Here's how the part is built. I have some questions about the finished solid (model axes, mm). A direction names the side the tool comes from. Coordinates: 2 decimals unless noted, no trailing zeros. Loops run counter-clockwise (first coordinate to the right, second up) from the corner with the lowest first, then second, coordinate; pieces in that order, holes last. Notation, with made-up numbers: (5.5, 0) - (16.5, 0) arc R12 cw to (16.5, 12) - close; hole circle Ø10 at (30.5, 33.5). An arc over 180 degrees is marked (long way). Use a Markdown table: item, result.
```python
from build123d import *

# Parameters (mm, degrees)
F0_W     = 90
F0_H     = 4
F1_DEPTH = 5
F2_R     = 1.661067913
F3_DEPTH = 3.5
F6_W     = 1.3
F6_H     = 4
F7_DEPTH = 1.3
F8_W     = 3.1040143222
F8_H     = 3.8397812168
F9_DEPTH = 89


# Not quite as in the source:
# - the program builds the solid bodies; features that only make, move or delete a surface that nothing else refers to are left out


with BuildPart() as f1:
    # F0 (on Top) → F1 (new body)
    with BuildSketch(Plane.XY):
        with Locations((9.9665279686, 16.8302931339)):
            Rectangle(F0_W, F0_H)
    extrude(amount=F1_DEPTH)

    # F2 (on face) → F3 (cut)
    with BuildSketch(Plane.XY.offset(5)):
        with Locations((-33.0299064517, 16.7948473245)):
            Circle(F2_R)
    extrude(amount=-F3_DEPTH, mode=Mode.SUBTRACT)

    # F6 (on face) → F7 (cut)
    with BuildSketch(Plane(origin=(0, 0, 0), x_dir=(1, 0, 0), z_dir=(0, 0, -1))):
        with Locations((6.5131389402, -16.8302931339)):
            Rectangle(F6_W, F6_H)
    extrude(amount=-F7_DEPTH, mode=Mode.SUBTRACT)

    # F8 (on face) → F9 (cut)
    with BuildSketch(Plane.YZ.offset(54.9665279686)):
        with Locations((16.8456220999, 2.3313869315)):
            Rectangle(F8_W, F8_H)
    extrude(amount=-F9_DEPTH, mode=Mode.SUBTRACT)


solid = f1.part
```
Q1. Please list where these lines run through material, in increasing order: L1, parallel to Z at x = 4, y = 16.2; L2, parallel to X at y = 17.6, z = 0.35; L3, parallel to Y at x = -11, z = 4.05. Write a range as from..to.
Check values:
| item | result |
|---|---|
| L1 | 0..0.41, 4.25..5 |
| L2 | -35.03..5.86, 7.16..54.97 |
| L3 | 14.83..15.29, 18.4..18.83 |
Q2. I want a section at B-B, the plane z = 2.4. Write out the boundary of the cut face in (x, y).
Check values:
| item | result |
|---|---|
| outline | (-35.03, 14.83) - (54.97, 14.83) - (54.97, 15.29) - (-32.32, 15.29) arc R1.66 cw to (-33.74, 15.29) - (-34.03, 15.29) - (-34.03, 15.47) arc R1.66 cw to (-34.03, 18.12) - (-34.03, 18.4) - (-33.47, 18.4) arc R1.66 cw to (-32.59, 18.4) - (54.97, 18.4) - (54.97, 18.83) - (-35.03, 18.83) - close |
Q3. Which directions (+Z, -Z, +X, -X, +Y, -Y) give clear straight access to the entire face, cutting with the end or side of a thin tool? Please do faces 4 (the face through (-14, 17, 0.411)), 5 (the face through (-35.033, 17, 2)).
Check values:
| item | result |
|---|---|
| face 4 | +X |
| face 5 | +Z, -Z, -X, +Y, -Y |
Q4. Will this pin go through, and if not, where does the flat tip stop? P1, Ø0.5, axis at x = -34.5, y = 16.5, coming from the +Z side.
Check values:
| item | result |
|---|---|
| P1 | z = 5 |
Q5. I want a section at A-A, the plane x = -6. Write out the boundary of the cut face in (y, z).
Check values:
| item | result |
|---|---|
| outline | (14.83, 0) - (18.83, 0) - (18.83, 5) - (14.83, 5) - close; hole (15.29, 0.41) - (18.4, 0.41) - (18.4, 4.25) - (15.29, 4.25) - close |
Q6. If we mould it in two halves opening along X, with no side actions, what happens to faces 1 (the face through (-34.033, 17, 1)), 2 (the face through (12, 17, 4.251)), 3 (the face through (-34.69, 16.87, 3.66))? For each: pulls with the +X half, pulls with the -X half, needs draft (parallel to the pull), parting line crosses it, or undercut.
Check values:
| item | result |
|---|---|
| face 1 | pulls with the +X half |
| face 2 | needs draft |
| face 3 | undercut |
